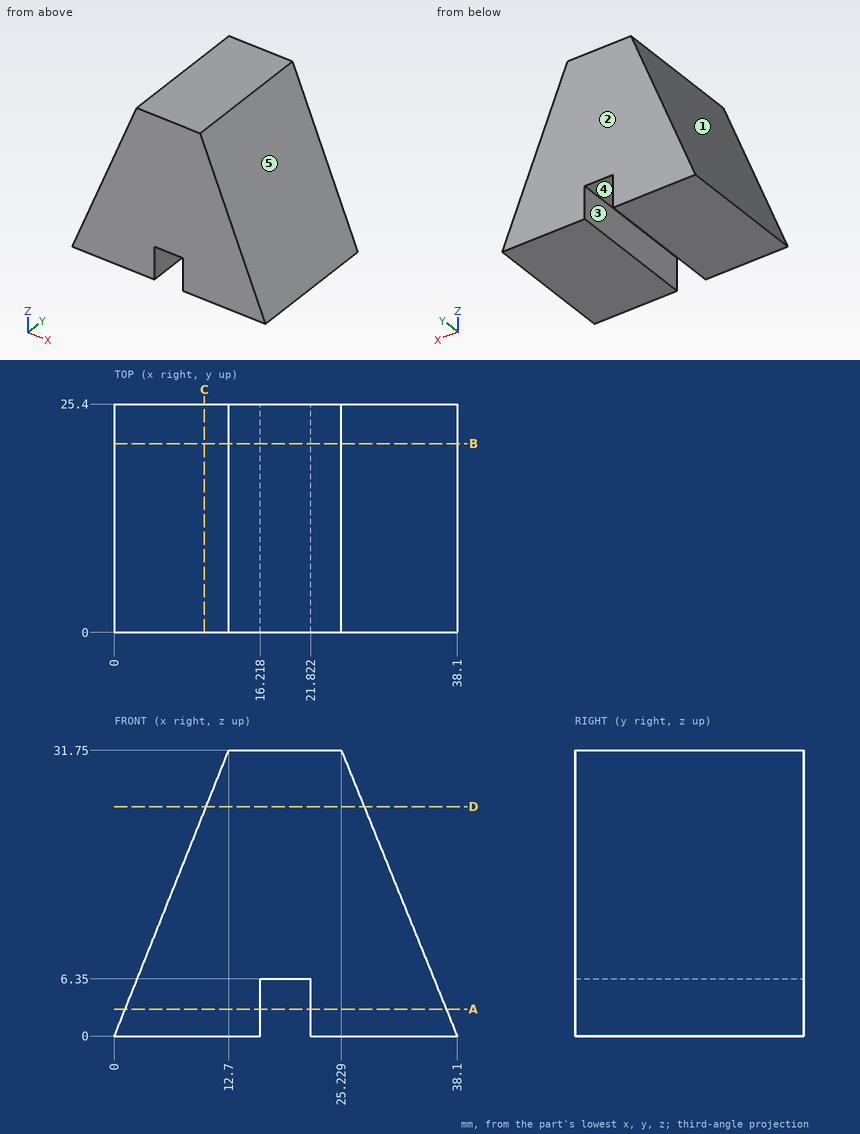
Part print with two shaded views. Sizes in mm from the minimum x, y, z corner. A direction names the side the tool comes from. Coordinates: 2 decimals unless noted, no trailing zeros. Order: outer loops, then holes, each group sorted by start corner. A loop starts at its lowest first (then second) coordinate and runs counter-clockwise, first axis right, second up.
(1) Mould opens along X. For the marked faces 1, 2 and 3 say: released by +X, released by -X, zero draft, split by the parting line, or undercut.
Solution:
face 1: released by -X
face 2: zero draft
face 3: undercut
(2) Saw through at A-A, the plane z = 3. Write the cut outline in (x, y).
Solution:
outline: (1.2, 0) - (16.22, 0) - (16.22, 25.4) - (1.2, 25.4) - close; (21.82, 0) - (36.88, 0) - (36.88, 25.4) - (21.82, 25.4) - close
(3) Which spindle directions (+Z, -Z, +X, -X, +Y, -Y) get a long thin tool onto all of the face, cutting with end or side? Do the marked faces 4 and 5. Say none if no direction does.
Solution:
face 4: -Z, +Y, -Y
face 5: +Z, +X, +Y, -Y
(4) Saw through at B-B, the plane y = 21. Write the cut outline in (x, z), and give its area (3 significant figures).
Solution:
outline: (0, 0) - (16.22, 0) - (16.22, 6.35) - (21.82, 6.35) - (21.82, 0) - (38.1, 0) - (25.23, 31.75) - (12.7, 31.75) - close
area: 768 mm2
(5) Drill centre lines: L1, parallel to Z at x = 21.5, y = 10.5; L2, parallel to X at y = 17, z = 3 (1 decimal); L3, parallel to X at y = 16, z = 4.5 (1 decimal). Where is each one in solid material? Low to high.
Solution:
L1: z = 6.35 to 31.75
L2: x = 1.2 to 16.2, 21.8 to 36.9
L3: x = 1.8 to 16.2, 21.8 to 36.3
(6) Pin check, flat tips, straight feed: pin 1 Ø12 at (y, z) = (15.5, 14.5) entering from +X (1 decimal); pin 2 Ø1.5 at (y, z) = (6, 14) entering from -X; pin 3 Ø1.9 at (y, z) = (9, 4) entering from -X; pin 4 Ø5 at (x, y) = (27.5, 5.5) entering from +Z. Stop position of each tip, or through.
Solution:
pin 1: stops at x = 34.7
pin 2: stops at x = 5.3
pin 3: stops at x = 1.22
pin 4: stops at z = 31.75
(7) Saw through at C-C, the plane x = 10. Write the cut outline in (y, z).
Solution:
outline: (0, 0) - (25.4, 0) - (25.4, 25) - (0, 25) - close
(8) Saw through at D-D, the plane z = 25.5. Write the cut outline in (x, y), and give its area (3 significant figures).
Solution:
outline: (10.2, 0) - (27.76, 0) - (27.76, 25.4) - (10.2, 25.4) - close
area: 446 mm2
